```python
from build123d import *

# Parameters (mm, degrees)
BOSS_EXTRUDE1_DEPTH     = 25
BOSS_EXTRUDE2_DEPTH     = 10
BOSS_EXTRUDE7_DEPTH     = 5
SKETCH4_R               = 9
BOSS_EXTRUDE4_DEPTH     = 2.5
BOSS_EXTRUDE6_DEPTH     = 25
SKETCH7_R               = 2
CUT_EXTRUDE1_DEPTH      = 12
FILLET1_R               = 10
CHAMFER1_SIZE           = 17.320508076
CHAMFER1_SIZE_2         = 10
CUT_EXTRUDE2_DEPTH      = 90.868306427
CUT_EXTRUDE2_DEPTH_BACK = 90.868306427
SKETCH9_R               = 3.25
SKETCH10_R              = 5.75
CUT_EXTRUDE3_DEPTH      = 111.143088753


# Some blends are built 0.0001 mm under size
with BuildPart() as part:
    # Sketch1 → Boss-Extrude1 (new, symmetric)
    with BuildSketch(Plane.XY):
        Polygon((25.5, -12.75), (25.5, -17.75), (-5, -17.75), (-5, 17.75), (25.5, 17.75), (25.5, 12.75), (0, 12.75), (0, -12.75), align=None)
    extrude(amount=BOSS_EXTRUDE1_DEPTH, both=True)

    # Sketch2 → Boss-Extrude2 (add, symmetric)
    with BuildSketch(Plane.XY):
        Polygon((-5, 17.75), (-5, 77.75), (5, 77.75), (25.5, 17.75), align=None)
        Polygon((5, -77.75), (-5, -77.75), (-5, -17.75), (25.5, -17.75), align=None)
    extrude(amount=BOSS_EXTRUDE2_DEPTH, both=True)

    # Sketch8 → Boss-Extrude7 (add)
    with BuildSketch(Plane.ZY.offset(5)):
        Polygon((10, 17.75), (25, 17.75), (25, -17.75), (10, -17.75), (10, -77.75), (-10, -77.75), (-10, -17.75), (-25, -17.75), (-25, 17.75), (-10, 17.75), (-10, 77.75), (10, 77.75), align=None)
    extrude(amount=BOSS_EXTRUDE7_DEPTH)

    # Sketch4 → Boss-Extrude4 (add)
    with BuildSketch(Plane.ZY.offset(10)):
        with Locations((0, 65)):
            Circle(SKETCH4_R)
        with Locations((0, -65)):
            Circle(SKETCH4_R)
    extrude(amount=BOSS_EXTRUDE4_DEPTH)

    # Sketch6 → Boss-Extrude6 (add)
    with BuildSketch(Plane.ZY.offset(12.5)):
        Polygon((7.332348419, 65), (3.666174209, 71.35), (-3.666174209, 71.35), (-7.332348419, 65), (-3.666174209, 58.65), (3.666174209, 58.65), align=None)
        Polygon((7.332348419, -65), (3.666174209, -58.65), (-3.666174209, -58.65), (-7.332348419, -65), (-3.666174209, -71.35), (3.666174209, -71.35), align=None)
    extrude(amount=BOSS_EXTRUDE6_DEPTH)

    # Sketch7 → Cut-Extrude1 (cut)
    with BuildSketch(Plane.ZY.offset(37.5)):
        with Locations((0, 65)):
            Circle(SKETCH7_R)
        with Locations((0, -65)):
            Circle(SKETCH7_R)
    extrude(amount=-CUT_EXTRUDE1_DEPTH, mode=Mode.SUBTRACT)

    # Fillet1
    fillet1_edges = [part.edges().sort_by_distance(p)[0] for p in [
        (-2.5, -77.75, -10),
        (-2.5, -77.75, 10),
        (-2.5, 77.75, -10),
        (-2.5, 77.75, 10),
    ]]
    fillet(fillet1_edges, radius=FILLET1_R - 0.0001)  # a hair under: the kernel refuses the full size

    # Chamfer1
    # the kernel refuses this chamfer: 17.320508076, 10 mm, written as the material it adds along each edge
    with BuildSketch(Plane(origin=(-10, 17.75, -10), x_dir=(0, 0.999813220622208, 0.019326765612700598), z_dir=(1, 0, 0))) as chamfer1_piece_1_section:
        Polygon((CHAMFER1_SIZE * 0.999813220604, -CHAMFER1_SIZE * 0.0193267656124), (-CHAMFER1_SIZE_2 * 0.0193267656127, -CHAMFER1_SIZE_2 * 0.999813220622), (0, 0), align=None)
    chamfer1_piece_1 = extrude(amount=35.5, mode=Mode.PRIVATE)
    chamfer1_piece_1 = split(chamfer1_piece_1, bisect_by=Plane(origin=(21.828322998, 28.496371714, -13.269268631), z_dir=(-0.9462910228001215, -0.32331609945670825, 0)), keep=Keep.TOP, mode=Mode.PRIVATE)
    add(chamfer1_piece_1)
    with BuildSketch(Plane(origin=(25.5, 17.75, 10), x_dir=(0, 0.9998132206222078, -0.019326765612700598), z_dir=(-1, 0, 0))) as chamfer1_piece_2_section:
        Polygon((CHAMFER1_SIZE * 0.999813220604, -CHAMFER1_SIZE * 0.0193267656124), (-CHAMFER1_SIZE_2 * 0.0193267656127, -CHAMFER1_SIZE_2 * 0.999813220622), (0, 0), align=None)
    chamfer1_piece_2 = extrude(amount=35.5, mode=Mode.PRIVATE)
    chamfer1_piece_2 = split(chamfer1_piece_2, bisect_by=Plane(origin=(21.828322998, 28.496371714, 13.269268631), z_dir=(-0.9462910228001215, -0.32331609945670825, 0)), keep=Keep.TOP, mode=Mode.PRIVATE)
    add(chamfer1_piece_2)
    with BuildSketch(Plane(origin=(25.5, -17.75, -10), x_dir=(0, -0.9998132206222078, 0.019326765612700598), z_dir=(-1, 0, 0))) as chamfer1_piece_3_section:
        Polygon((CHAMFER1_SIZE * 0.999813220604, -CHAMFER1_SIZE * 0.0193267656124), (-CHAMFER1_SIZE_2 * 0.0193267656127, -CHAMFER1_SIZE_2 * 0.999813220622), (0, 0), align=None)
    chamfer1_piece_3 = extrude(amount=35.5, mode=Mode.PRIVATE)
    chamfer1_piece_3 = split(chamfer1_piece_3, bisect_by=Plane(origin=(21.828322998, -28.496371714, -13.269268631), z_dir=(-0.9462910228001215, 0.32331609945670825, 0)), keep=Keep.TOP, mode=Mode.PRIVATE)
    add(chamfer1_piece_3)
    with BuildSketch(Plane(origin=(-10, -17.75, 10), x_dir=(0, -0.999813220622208, -0.019326765612700695), z_dir=(1, 0, 0))) as chamfer1_piece_4_section:
        Polygon((CHAMFER1_SIZE * 0.999813220604, -CHAMFER1_SIZE * 0.0193267656124), (-CHAMFER1_SIZE_2 * 0.0193267656127, -CHAMFER1_SIZE_2 * 0.999813220622), (0, 0), align=None)
    chamfer1_piece_4 = extrude(amount=35.5, mode=Mode.PRIVATE)
    chamfer1_piece_4 = split(chamfer1_piece_4, bisect_by=Plane(origin=(21.828322998, -28.496371714, 13.269268631), z_dir=(-0.9462910228001215, 0.32331609945670825, 0)), keep=Keep.TOP, mode=Mode.PRIVATE)
    add(chamfer1_piece_4)

    # Sketch9 → Cut-Extrude2 (cut, two sides: drawn at the far end of the back side and taken through both)
    with BuildSketch(Plane(origin=(0, 0, 0), x_dir=(1, 0, 0), z_dir=(0, 1, 0)).offset(-CUT_EXTRUDE2_DEPTH_BACK)):
        with Locations((12.75, 0)):
            Circle(SKETCH9_R)
    extrude(amount=CUT_EXTRUDE2_DEPTH + CUT_EXTRUDE2_DEPTH_BACK, mode=Mode.SUBTRACT)

    # Sketch10 → Cut-Extrude3 (cut, through all)
    with BuildSketch(Plane(origin=(0, -22.75, 0), x_dir=(1, 0, 0), z_dir=(0, 1, 0))):
        with Locations(Location((12.75, 0, 0), (0, 0, 180))):
            Circle(SKETCH10_R)
    cut_extrude3 = extrude(amount=-CUT_EXTRUDE3_DEPTH, mode=Mode.SUBTRACT)

    # Mirror1: Cut-Extrude3 across plane
    add(cut_extrude3.mirror(Plane.ZX), mode=Mode.SUBTRACT)


solid = part.part
```
Geometry check sheet. Reference: the model listing, model coordinates, mm. A direction names the side the tool comes from. Give positions to 0.01 mm unless a question says otherwise; leave off trailing zeros. Loops run counter-clockwise (first coordinate to the right, second up) from the corner with the lowest first, then second, coordinate; pieces in that order, holes last. Notation, with made-up numbers: M 26,88 L 31,88 A23 cw 31,118 Z; hole C 74.25,65.25 d3. An arc over 180 degrees is marked long. Write item = value, one per line. Start each with the question number.
1. Go/stop test with flat-tipped pins: P1, Ø6, axis at x = -26.5, z = 0.5, coming from the +Y side; P2, Ø10.5, axis at x = 12.75, z = 0, coming from the -Y side; P3, Ø4, axis at x = 8, z = -21.5, coming from the +Y side; P4, Ø5, axis at x = 12.75, z = 0, coming from the +Y side. Record where each tip stops, or that it passes through.
2. Section check D-D, the plane y = 7. Enter the section's corners in (x, z), plus the area to 3 significant figures.
3. Section check A-A, the plane x = -31.5. Enter the section's corners in (y, z).
4. Section check C-C, the plane z = -13. Enter the section's corners in (x, y).
5. Tool access check on faces 4 (the face through (10, 22.75, -2)), 5 (the face through (8, 17.75, -23)), 6 (the face through (-11.232, 56.214, -1.951)), 7 (the face through (-24.825, -61.869, 5.525)). Record the directions out of +Z, -Z, +X, -X, +Y, -Y that give a thin tool (end or side, any length) a straight path to the whole face; none if there is none.
6. Thickness scan on probe 1 along Y at (x, z) = (-17.5, 0); probe 2 along Y at (x, z) = (-33, 0); probe 3 along Y at (x, z) = (8, 2.5). Record the ranges inside material, lowest first.
7. Section check B-B, the plane y = 26.5. Enter the section's corners in (x, z), plus the area to 3 significant figures.
8. Draft check along Y on faces 1 (the face through (8, 26.53, 14.93)), 2 (the face through (-10, -1, 0)), 3 (the face through (-4, 0, -25)). Enter one of: +Y half, -Y half, draft (parallel to the pull), parting line (faces both ways), or undercut.
Values follow:
q1.P1 = 71.35
q1.P2 = -22.75
q1.P3 = 18.62
q1.P4 = through
q2.outline = M -10,-25 L 0,-25 L 0,25 L -10,25 Z
q2.area = 500 mm^2
q3.outline = M -71.35,-3.67 L -65,-7.33 L -58.65,-3.67 L -58.65,3.67 L -65,7.33 L -71.35,3.67 Z; M 58.65,-3.67 L 65,-7.33 L 71.35,-3.67 L 71.35,3.67 L 65,7.33 L 58.65,3.67 Z; hole C -65,0 d4; hole C 65,0 d4
q4.outline = M -10,-29.87 L 21.36,-29.87 L 25.5,-17.75 L 25.5,-12.75 L 0,-12.75 L 0,12.75 L 25.5,12.75 L 25.5,17.75 L 21.36,29.87 L -10,29.87 Z
q5.face_4 = +Y
q5.face_5 = -Z, +X, -X, +Y
q5.face_6 = -X
q5.face_7 = +Z, -X
q6.probe_1 = -71.35 to -58.65, 58.65 to 71.35
q6.probe_2 = -71.35 to -67, -63 to -58.65, 58.65 to 63, 67 to 71.35
q6.probe_3 = -22.75 to -12.75, 12.75 to 22.75
q7.outline = M -10,-14.95 L 22.51,-14.95 L 22.51,14.95 L -10,14.95 Z; hole C 12.75,0 d11.5
q7.area = 868 mm^2
q8.face_1 = +Y half
q8.face_2 = undercut
q8.face_3 = draft
